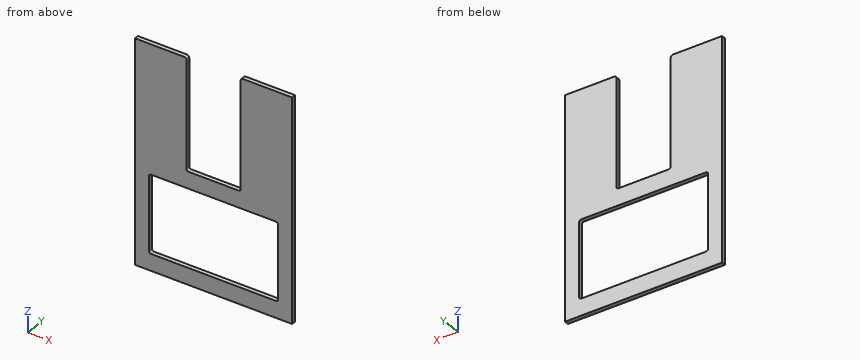
from build123d import *

# Parameters (mm, degrees)
SKETCH1_W           = 146.05
SKETCH1_H           = 88.9
BOSS_EXTRUDE1_DEPTH = 4.7625
FILLET1_R           = 2.54


with BuildPart() as part:
    # Sketch1 → Boss-Extrude1 (new body)
    with BuildSketch(Plane(origin=(0, 0, 0), x_dir=(1, 0, 0), z_dir=(0, 1, 0))):
        Polygon((-30.734, -127), (-30.734, 0), (30.734, 0), (30.734, -127), (88.9, -127), (88.9, 127), (-88.9, 127), (-88.9, -127), align=None)
        with Locations((0, 63.5)):
            Rectangle(SKETCH1_W, SKETCH1_H, mode=Mode.SUBTRACT)
    extrude(amount=BOSS_EXTRUDE1_DEPTH)

    # Fillet1
    fillet1_edges = [part.edges().sort_by_distance(p)[0] for p in [
        (30.734, 2.38125, 127),
        (30.734, 2.38125, 0),
        (-30.734, 2.38125, 0),
        (-30.734, 2.38125, 127),
        (-73.025, 2.38125, -107.95),
        (-73.025, 2.38125, -19.05),
        (73.025, 2.38125, -19.05),
        (73.025, 2.38125, -107.95),
    ]]
    fillet(fillet1_edges, radius=FILLET1_R)


solid = part.part
Can you work these out from the model? Positions are in its coordinate system, mm. Round coordinates to 2 decimals unless told otherwise and drop trailing zeros. Write each loop counter-clockwise with the first axis right and the second up, starting at its lowest first coordinate (ties: lowest second). Pieces come first, ordered by that corner, then holes. Notation, with made-up numbers: (73, -12) - (82, -12) arc R20 cw to (82, 8) - close; hole circle Ø4 at (66.25, 42.5). An arc over 180 degrees is marked (long way). Write each question's results on one line, items separated by ' | '. Start each with the question number.
1) Please list where these lines run through material, in increasing order: line 1 (X direction, y = 2.4, z = 97.5); line 2 (Z direction, x = 16.5, y = 4.2); line 3 (X direction, y = 1.5, z = -24) (3 decimals).
2) Suppose I cut it at B-B (z = -96). List the corners of the cut face in (x, y) for me (1 decimal), and give its area (3 significant figures).
3) Suppose I cut it at C-C (y = 1.45). List the corners of the cut face in (x, z) for me (3 decimals).
4) For pin 1 Ø1 at (x, y) = (29, 1.5) entering from +Z; pin 2 Ø2.5 at (x, y) = (-4, 1.5) entering from +Z, each with a flat end and sliding along its axis, tell me the tip position at first contact or that it passes through.
5) Suppose I cut it at A-A (x = 43). List the corners of the cut face in (y, z) for me.
Here are the results:
1) line 1: x = -88.9 to -30.73, 30.73 to 88.9 | line 2: z = -127 to -107.95, -19.05 to 0 | line 3: x = -88.9 to -73.025, 73.025 to 88.9
2) outline: (-88.9, 0) - (-73, 0) - (-73, 4.8) - (-88.9, 4.8) - close; (73, 0) - (88.9, 0) - (88.9, 4.8) - (73, 4.8) - close | area: 151 mm2
3) outline: (-88.9, -127) - (88.9, -127) - (88.9, 127) - (33.274, 127) arc R2.54 ccw to (30.734, 124.46) - (30.734, 2.54) arc R2.54 cw to (28.194, 0) - (-28.194, 0) arc R2.54 cw to (-30.734, 2.54) - (-30.734, 124.46) arc R2.54 ccw to (-33.274, 127) - (-88.9, 127) - close; hole (-73.025, -105.41) arc R2.54 ccw to (-70.485, -107.95) - (70.485, -107.95) arc R2.54 ccw to (73.025, -105.41) - (73.025, -21.59) arc R2.54 ccw to (70.485, -19.05) - (-70.485, -19.05) arc R2.54 ccw to (-73.025, -21.59) - close
4) pin 1: stops at z = 0.36 | pin 2: stops at z = 0
5) outline: (0, -127) - (4.76, -127) - (4.76, -107.95) - (0, -107.95) - close; (0, -19.05) - (4.76, -19.05) - (4.76, 127) - (0, 127) - close
